```python
from build123d import *

# Parameters (mm, degrees)
F0_W     = 29.5
F0_H     = 12.75
F0_W_2   = 20
F0_W_3   = 15
F0_H_2   = 12.25
F1_DEPTH = 12.5
F2_DEPTH = 27.5
F4_DEPTH = 15
F6_R     = 0.99999


# Not quite as in the source:
# - a fillet or chamfer is up to 0.001 mm smaller than in the source, because OpenCascade refuses the exact size


with BuildPart() as f1:
    # F0 (on Top) → F1 (new body)
    with BuildSketch(Plane.XY):
        with Locations((-14.75, -6.375)):
            Rectangle(F0_W, F0_H)
        Polygon((20, -12.75), (0, -12.75), (-29.5, -12.75), (-29.5, -14.75), (0, -14.75), (20, -25), align=None)
        with Locations((10, -6.375)):
            Rectangle(F0_W_2, F0_H)
        with Locations((27.5, -6.375)):
            Rectangle(F0_W_3, F0_H)
        with Locations((27.5, -18.875)):
            Rectangle(F0_W_3, F0_H_2)
    extrude(amount=F1_DEPTH)

    # F0 (on Top) → F2 (join)
    with BuildSketch(Plane.XY):
        Polygon((20, -12.75), (0, -12.75), (-29.5, -12.75), (-29.5, -14.75), (0, -14.75), (20, -25), align=None)
        with Locations((27.5, -18.875)):
            Rectangle(F0_W_3, F0_H_2)
    extrude(amount=F2_DEPTH)

    # F3 (on face) → F4 (cut)
    with BuildSketch(Plane.YZ.offset(35)):
        Polygon((-25, 2), (0, 2), (0, 12.5), (-12.75, 12.5), (-25, 12.5), align=None)
    extrude(amount=-F4_DEPTH, mode=Mode.SUBTRACT)

    # F5: F1 across plane


with BuildPart() as f1_1:
    add(f1.part)
    add(f1.part.mirror(Plane.XZ))

    # F6 (radius 1 in the source; OpenCascade refuses exactly that, so slightly less here)
    f6_edges = [f1_1.edges().sort_by_distance(p)[0] for p in [
        (-14.75, -14.75, 0),
        (10, -19.875, 0),
        (27.5, -25, 0),
        (35, 0, 0),
        (27.5, 25, 0),
        (10, 19.875, 0),
        (-14.75, 14.75, 0),
        (-29.5, 0, 0),
        (-29.5, -13.75, 27.5),
        (-14.75, -14.75, 27.5),
        (10, -19.875, 27.5),
        (27.5, -25, 27.5),
        (35, -18.875, 27.5),
        (2.75, -12.75, 27.5),
        (-29.5, 13.75, 27.5),
        (-14.75, 14.75, 27.5),
        (10, 19.875, 27.5),
        (27.5, 25, 27.5),
        (35, 18.875, 27.5),
        (2.75, 12.75, 27.5),
        (35, 25, 20),
        (35, 18.875, 12.5),
        (35, 12.75, 20),
        (35, -18.875, 12.5),
        (35, -12.75, 20),
        (35, -25, 20),
        (-29.5, 0, 12.5),
    ]]
    fillet(f6_edges, radius=F6_R)


solid = f1_1.part
```
The model under review builds one solid part; all positions refer to its coordinate system, in mm. A direction names the side the tool comes from. Give positions to 0.01 mm unless a question says otherwise; leave off trailing zeros. Loops run counter-clockwise (first coordinate to the right, second up) from the corner with the lowest first, then second, coordinate; pieces in that order, holes last. Notation, with made-up numbers: (39, -4) -> (96, -4) arc R19 ccw to (96, 21) -> close; hole circle Ø7 at (35, 77). An arc over 180 degrees is marked (long way). Use CSV: the item, a comma, the result in double quotes.
1. Consider section D-D, the plane z = 10.25. Write out the cut boundary in (x, y), then the cut area to 3 significant figures.
Result:
outline,"(-29.5, -14.75) -> (0, -14.75) -> (20, -25) -> (20, 25) -> (0, 14.75) -> (-29.5, 14.75) -> close"
area,"1,670 mm²"
2. Consider section C-C, the plane y = -5.5. Write out the cut boundary in (x, z).
Result:
outline,"(-29.5, 1) arc R1 ccw to (-28.5, 0) -> (34, 0) arc R1 ccw to (35, 1) -> (35, 2) -> (20, 2) -> (20, 12.5) -> (-28.5, 12.5) arc R1 ccw to (-29.5, 11.5) -> close"
3. Consider section A-A, the plane z = 18.75. Write out the cut boundary in (x, y).
Result:
outline,"(-29.5, -14.75) -> (0, -14.75) -> (20, -25) -> (34, -25) arc R1 ccw to (35, -24) -> (35, -13.75) arc R1 ccw to (34, -12.75) -> (-29.5, -12.75) -> close; (-29.5, 12.75) -> (34, 12.75) arc R1 ccw to (35, 13.75) -> (35, 24) arc R1 ccw to (34, 25) -> (20, 25) -> (0, 14.75) -> (-29.5, 14.75) -> close"
4. The part is to be moulded in two halves that separate along Z. For faces 1 (the face through (20, 0, 7)), 2 (the face through (23, 18, 27.5)), 3 (the face through (27, 25, 19)), say which applies: +Z half, -Z half, draft (parallel to the pull), parting line (faces both ways), or undercut.
Result:
face 1,"undercut"
face 2,"+Z half"
face 3,"draft"
5. Machinability: for faces 4 (the face through (-15, -14.75, 14)), 5 (the face through (28, 0, 2)), 6 (the face through (-5, 0, 12.5)), 7 (the face through (35, -19, 20)), 8 (the face through (10.164, -19.639, 27.199)), which of the approach directions +Z, -Z, +X, -X, +Y, -Y give a long, thin tool a straight path to every point of the face, cutting with its end or side? Answer none if there is none.
Result:
face 4,"+Z, -Z, -X, -Y"
face 5,"+X, +Y, -Y"
face 6,"+Z, +X, -X"
face 7,"+Z, -Z, +X, +Y, -Y"
face 8,"+Z, -X, -Y"
6. For P1, Ø7.5, axis at x = -8.5, z = 11, coming from the -Y side; P2, Ø4, axis at x = 0, z = 10.5, coming from the +Y side (3 decimals); P3, Ø3, axis at y = -5, z = 8.5, coming from the +X side; P4, Ø8.5, axis at y = 6.5, z = 5, coming from the +X side, all flat-tipped, find the tip position at first contact; note any pin that passes through.
Result:
P1,"stops at y = -14.75"
P2,"stops at y = 15.775"
P3,"stops at x = 20"
P4,"stops at x = 35"
7. To check wall thickness, follow probe 1 along Y at (x, z) = (20, 15.75); probe 2 along Z at (x, y) = (26.5, -19); probe 3 along Y at (x, z) = (-11.5, 17.75). State the ranges of each line that lie inside material, in increasing order. Write a range as from..to.
Result:
probe 1,"y = -25..-12.75, 12.75..25"
probe 2,"z = 0..2, 12.5..27.5"
probe 3,"y = -14.75..-12.75, 12.75..14.75"
